```python
from build123d import *

# Parameters (mm, degrees)
SKETCH_1_R          = 5
EXTRUDE_1_DEPTH     = 19
SKETCH_3_R          = 3.1
CUT_EXTRUDE_1_DEPTH = 17
EXTRUDE_2_DEPTH     = 12
SKETCH_8_R          = 3.95
EXTRUDE_4_DEPTH     = 5.5
SKETCH_9_R          = 2.725
CUT_EXTRUDE_2_DEPTH = 5.5
EXTRUDE_5_DEPTH     = 4
FILLET_1_R          = 0.2
CHAMFER_1_SIZE      = 0.5
CHAMFER_2_SIZE      = 0.4
CHAMFER_3_SIZE      = 0.2


with BuildPart() as part:
    # 草图1 → 凸台-拉伸1 (new body)
    with BuildSketch(Plane(origin=(0, 0, 0), x_dir=(0, 0, -1), z_dir=(1, 0, 0))):
        Circle(SKETCH_1_R)
    extrude(amount=EXTRUDE_1_DEPTH)

    # 草图3 → 切除-拉伸1 (cut)
    with BuildSketch(Plane(origin=(19, 0, 0), x_dir=(0, 0, -1), z_dir=(1, 0, 0))):
        Circle(SKETCH_3_R)
    extrude(amount=-CUT_EXTRUDE_1_DEPTH, mode=Mode.SUBTRACT)

    # 草图5 → 凸台-拉伸2 (add)
    with BuildSketch(Plane(origin=(2, 0, 0), x_dir=(0, 0, -1), z_dir=(1, 0, 0))):
        with BuildLine():
            Line((-1.688194302, 2.6), (1.688194302, 2.6))
            Line((1.688194302, 2.6), (1.688194302, 5.234500931))
            ThreePointArc((1.688194302, 5.234500931), (0, 5.5), (-1.688194302, 5.234500931))
            Line((-1.688194302, 5.234500931), (-1.688194302, 2.6))
        make_face()
    extrude(amount=EXTRUDE_2_DEPTH)

    # 草图8 → 凸台-拉伸4 (add)
    with BuildSketch(Plane.ZY):
        Circle(SKETCH_8_R)
    extrude(amount=EXTRUDE_4_DEPTH)

    # 草图9 → 切除-拉伸2 (cut)
    with BuildSketch(Plane.ZY.offset(5.5)):
        Circle(SKETCH_9_R)
    extrude(amount=-CUT_EXTRUDE_2_DEPTH, mode=Mode.SUBTRACT)

    # 草图10 → 凸台-拉伸5 (add)
    with BuildSketch(Plane.ZY):
        Polygon((0.721687836, 1.25), (-0.721687836, 1.25), (-1.443375673, 0), (-0.721687836, -1.25), (0.721687836, -1.25), (1.443375673, 0), align=None)
    extrude(amount=EXTRUDE_5_DEPTH)

    # 圆角1
    fillet_1_edges = [part.edges().sort_by_distance(p)[0] for p in [
        (8, 4.70637865, 1.688194302),
        (8, 5.234500931, 1.688194302),
        (8, 4.70637865, -1.688194302),
        (8, 5.234500931, -1.688194302),
    ]]
    fillet(fillet_1_edges, radius=FILLET_1_R)

    # 倒角1
    # the kernel refuses this chamfer: 0.5 mm, written as the material it takes off along each edge
    with BuildSketch(Plane(origin=(14, 0, 0), x_dir=(0, 0.8686030413593419, -0.4955085837211114), z_dir=(0, -0.4955085837211114, -0.8686030413593419))) as chamfer_1_piece_1:
        Polygon((5.5, -CHAMFER_1_SIZE), (5.5 - CHAMFER_1_SIZE, 0), (5.5, 0), align=None)
    revolve(axis=Axis((14, 0, 0), (1, 0, 0)), revolution_arc=59.40658503, mode=Mode.SUBTRACT)
    with BuildSketch(Plane(origin=(2, 0, 0), x_dir=(0, 0.8686030413593415, -0.4955085837211117), z_dir=(0, -0.4955085837211117, -0.8686030413593415))) as chamfer_1_piece_2:
        Polygon((5.5 - CHAMFER_1_SIZE, 0), (5.5, CHAMFER_1_SIZE), (5.5, 0), align=None)
    revolve(axis=Axis((2, 0, 0), (1, 0, 0)), revolution_arc=59.40658503, mode=Mode.SUBTRACT)
    with BuildSketch(Plane(origin=(14, 2.6, 2.974035796), x_dir=(0.027495876610585623, 0.9996219169112968, 0), z_dir=(0, 0, -1))) as chamfer_1_piece_3_section:
        Polygon((CHAMFER_1_SIZE * 0.999621916911, -CHAMFER_1_SIZE * 0.0274958766106), (-CHAMFER_1_SIZE * 0.0274958766106, -CHAMFER_1_SIZE * 0.999621916911), (0, 0), align=None)
    chamfer_1_piece_3 = extrude(amount=5.948071591, mode=Mode.PRIVATE)
    chamfer_1_piece_3 = chamfer_1_piece_3 & Plane(origin=(13.821912141, 0, 0), x_dir=(0, 0, -1), z_dir=(1, 0, 0)) * Cylinder(3.1, 14, mode=Mode.PRIVATE)
    add(chamfer_1_piece_3, mode=Mode.SUBTRACT)

    # 倒角2
    chamfer_2_edges = [part.edges().sort_by_distance(p)[0] for p in [
        (19, 0, 3.1),
    ]]
    chamfer(chamfer_2_edges, length=CHAMFER_2_SIZE)

    # 倒角3
    chamfer_3_edges = [part.edges().sort_by_distance(p)[0] for p in [
        (-5.5, 0, -3.95),
        (-5.5, 0, -2.725),
        (-4, 0.625, 1.082531755),
        (-4, 1.25, 0),
        (-4, 0.625, -1.082531755),
        (-4, -0.625, -1.082531755),
        (-4, -1.25, 0),
        (-4, -0.625, 1.082531755),
    ]]
    chamfer(chamfer_3_edges, length=CHAMFER_3_SIZE)


solid = part.part
```
Design review of the part built by this model. Coordinates are the model's own, in mm. A direction names the side the tool comes from. Give positions to 0.01 mm unless a question says otherwise; leave off trailing zeros. Write each loop counter-clockwise with the first axis right and the second up, starting at its lowest first coordinate (ties: lowest second). Pieces come first, ordered by that corner, then holes. Notation, with made-up numbers: (57.25, 79.25) - (77.25, 79.25) arc R22 cw to (77.25, 111.25) - close; hole circle Ø9 at (-1, -19). An arc over 180 degrees is marked (long way). Return JSON: item names as keys, results as strings. Group by question number.
(1) Insertion check: pin 1 (5 mm diameter, centred on y = 0, z = 0, fed in from -X); pin 2 (1.6 mm diameter, centred on x = -2, z = 0.5, fed in from +Y); pin 3 (3 mm diameter, centred on x = 11, z = 3, fed in from +Y). Each pin has a flat end and moves straight along its axis. Give the tip position at first contact, or say it passes through.
(2) To check wall thickness, follow probe 1 along Y at (x, z) = (12.75, 0); probe 2 along X at (y, z) = (-3.5, 3.5); probe 3 along Z at (x, y) = (10.25, -2). State the ranges of each line that lie inside material, in increasing order.
(3) Machinability: for faces 5 (the flat face through (-4, 0, 0)), 6 (the cylindrical face through (7.9, 5.5, 0)), which of the approach directions +Z, -Z, +X, -X, +Y, -Y give a long, thin tool a straight path to every point of the face, cutting with its end or side? Answer none if there is none.
(4) We need section C-C, the plane x = 0.5. Give the boundary of the cut face in (y, z), then the cut area to 3 significant figures.
(5) We need section A-A, the plane x = 10.5. Give the boundary of the cut face in (y, z), then the cut area to 3 significant figures.
(6) Mouldability with a two-part tool opening along Z and no side actions: class faces 1 (the flat face through (-1.87, -0.63, 1.08)), 2 (the flat face through (-1.873, 0.616, 1.088)), 3 (the flat face through (0, 2, -4)), 4 (the cylindrical face through (9.37, -4.88, 1.08)) as +Z half, -Z half, draft (parallel to the pull), parting line (faces both ways), or undercut.
Reported:
{
 "1": {"pin 1": "stops at x = -4", "pin 2": "stops at y = 3.95", "pin 3": "stops at y = 5.29"},
 "2": {"probe 1": "y = -5 to -3.1, 2.6 to 5.5", "probe 2": "x = 0 to 19", "probe 3": "z = -4.58 to -2.37, 2.37 to 4.58"},
 "3": {"face 5": "-X", "face 6": "+X, -X, +Y"},
 "4": {"outline": "circle Ø10 at (0, 0)", "area": "78.5 mm2"},
 "5": {"outline": "(4.66, -1.82) arc R0.2 cw to (4.85, -1.69) - (5.09, -1.69) arc R0.2 ccw to (5.28, -1.54) arc R5.5 ccw to (5.28, 1.54) arc R0.2 ccw to (5.09, 1.69) - (4.85, 1.69) arc R0.2 cw to (4.66, 1.82) arc R5 ccw (long way) to start; hole (2.6, -1.69) - (2.6, 1.69) arc R3.1 ccw (long way) to start", "area": "51.2 mm2"},
 "6": {"face 1": "undercut", "face 2": "undercut", "face 3": "draft", "face 4": "parting line"}
}
